The listing builds one solid part. Answer for the finished solid, in the listing's coordinates (mm). Round coordinates to 2 decimals unless told otherwise and drop trailing zeros. Write each loop counter-clockwise with the first axis right and the second up, starting at its lowest first coordinate (ties: lowest second). Pieces come first, ordered by that corner, then holes. Notation, with made-up numbers: M -34,13 L 2,13 A35 ccw 2,46 Z; hole C -23.75,53.25 d10. An arc over 180 degrees is marked long. One line per item, written item: value. Start each with the question number.
(1) Given P1, Ø1, axis at y = 2, z = -168, coming from the +X side; P2, Ø1.9, axis at x = 7.5, z = -222.3, coming from the +Y side; P3, Ø1.5, axis at x = 36, y = 2, coming from the +Z side, each flat-ended and moving along its own axis, determine where each tip first touches the part or whether it passes through.
(2) Consider probe 1 along Z at (x, y) = (145, 0.8); probe 2 along X at (y, z) = (2.15, -171.5); probe 3 along Z at (x, y) = (70, 2.45). Determine where each line is inside the solid, lowest interval first.
(3) For a pull along X with two mould halves and no side action, classify faces 1 (the cylindrical face through (3.01, 1.52, -2.85)), 2 (the cylindrical face through (167.15, 1.52, -3.01)), 3 (the flat face through (83, 3, -158)) as released by +X, released by -X, zero draft, split by the parting line, or undercut.
(4) Section C-C (y = 1.5) is taken. State how many separate pieces and enclosed holes the cut face has, plus the area to 3 significant figures.
(5) Section B-B (z = -149) is taken. Determine the outline of the cut face in (x, y).
(6) Section A-A (x = 179) is taken. Determine the outline of the cut face in (y, z).
```python
from build123d import *

# Parameters (mm, degrees)
BOSS_EXTRUDE1_DEPTH = 3
FILLET1_R           = 200
FILLET2_R           = 10
CUT_EXTRUDE2_DEPTH  = 429.345808882
SKETCH3_W           = 42
SKETCH3_H           = 23
SKETCH3_H_2         = 19
CUT_EXTRUDE3_DEPTH  = 429.345808882
SKETCH4_R           = 1.6
CUT_EXTRUDE5_DEPTH  = 429.345808882
SKETCH5_R           = 1.6
CUT_EXTRUDE6_DEPTH  = 429.345808882
SKETCH6_W           = 66
SKETCH6_H           = 15
SKETCH6_R           = 1.6
BOSS_EXTRUDE2_DEPTH = 3
FILLET3_R           = 5
SKETCH7_R           = 1.6
CUT_EXTRUDE7_DEPTH  = 435.224748243
SKETCH9_R           = 1.6
CUT_EXTRUDE8_DEPTH  = 435.224748243
SKETCH10_W          = 280
SKETCH10_H          = 108.680633212
CUT_EXTRUDE9_DEPTH  = 10


with BuildPart() as part:
    # Sketch1 → Boss-Extrude1 (new body)
    with BuildSketch(Plane(origin=(0, 0, 0), x_dir=(1, 0, 0), z_dir=(0, 1, 0))):
        Polygon((0, 0), (170, 0), (170, 300), (225, 300), (225, 367.51288694), (85, 330), (-55, 367.51288694), (-55, 300), (0, 300), align=None)
    extrude(amount=BOSS_EXTRUDE1_DEPTH)

    # Fillet1
    fillet1_edges = [part.edges().sort_by_distance(p)[0] for p in [
        (85, 1.5, -330),
    ]]
    fillet(fillet1_edges, radius=FILLET1_R)

    # Fillet2
    fillet2_edges = [part.edges().sort_by_distance(p)[0] for p in [
        (0, 1.5, -300),
        (-55, 1.5, -300),
        (-55, 1.5, -367.51288694),
        (225, 1.5, -367.51288694),
        (225, 1.5, -300),
        (170, 1.5, -300),
        (170, 1.5, 0),
        (0, 1.5, 0),
    ]]
    fillet(fillet2_edges, radius=FILLET2_R)

    # Sketch2 → Cut-Extrude2 (cut, through all)
    with BuildSketch(Plane(origin=(0, 3, 0), x_dir=(1, 0, 0), z_dir=(0, 1, 0))):
        with BuildLine():
            ThreePointArc((132.5, 80), (118.587572106, 113.587572106), (85, 127.5))
            Line((85, 127.5), (85, 32.5))
            ThreePointArc((85, 32.5), (118.587572106, 46.412427894), (132.5, 80))
        make_face()
        with BuildLine():
            Line((85, 32.5), (85, 127.5))
            ThreePointArc((85, 127.5), (37.5, 80), (85, 32.5))
        make_face()
    extrude(amount=-CUT_EXTRUDE2_DEPTH, mode=Mode.SUBTRACT)

    # Sketch3 → Cut-Extrude3 (cut, through all)
    with BuildSketch(Plane(origin=(0, 3, 0), x_dir=(1, 0, 0), z_dir=(0, 1, 0))):
        with Locations((40, 267.3)):
            Rectangle(SKETCH3_W, SKETCH3_H)
        with Locations((130, 267.3)):
            Rectangle(SKETCH3_W, SKETCH3_H)
        with Locations((40, 9.5)):
            Rectangle(SKETCH3_W, SKETCH3_H_2)
        with Locations((130, 9.5)):
            Rectangle(SKETCH3_W, SKETCH3_H_2)
    extrude(amount=-CUT_EXTRUDE3_DEPTH, mode=Mode.SUBTRACT)

    # Sketch4 → Cut-Extrude5 (cut, through all)
    with BuildSketch(Plane(origin=(0, 3, 0), x_dir=(1, 0, 0), z_dir=(0, 1, 0))):
        with Locations(Location((85, 133, 0), (0, 0, 270))):
            Circle(SKETCH4_R)
        with Locations(Location((122.476659403, 117.476659403, 0), (0, 0, 270))):
            Circle(SKETCH4_R)
        with Locations(Location((138, 80, 0), (0, 0, 270))):
            Circle(SKETCH4_R)
        with Locations(Location((122.476659403, 42.523340597, 0), (0, 0, 270))):
            Circle(SKETCH4_R)
        with Locations(Location((85, 27, 0), (0, 0, 270))):
            Circle(SKETCH4_R)
        with Locations(Location((47.523340597, 42.523340597, 0), (0, 0, 270))):
            Circle(SKETCH4_R)
        with Locations(Location((32, 80, 0), (0, 0, 270))):
            Circle(SKETCH4_R)
        with Locations(Location((47.523340597, 117.476659403, 0), (0, 0, 270))):
            Circle(SKETCH4_R)
    extrude(amount=-CUT_EXTRUDE5_DEPTH, mode=Mode.SUBTRACT)

    # Sketch5 → Cut-Extrude6 (cut, through all)
    with BuildSketch(Plane(origin=(0, 3, 0), x_dir=(1, 0, 0), z_dir=(0, 1, 0))):
        with Locations(Location((7.5, 312, 0), (0, 0, 270))):
            Circle(SKETCH5_R)
        with Locations(Location((7.5, 267.3, 0), (0, 0, 270))):
            Circle(SKETCH5_R)
        with Locations(Location((7.5, 222.3, 0), (0, 0, 270))):
            Circle(SKETCH5_R)
        with Locations(Location((7.5, 97.5, 0), (0, 0, 270))):
            Circle(SKETCH5_R)
        with Locations(Location((7.5, 7.5, 0), (0, 0, 270))):
            Circle(SKETCH5_R)
        with Locations(Location((7.5, 52.5, 0), (0, 0, 270))):
            Circle(SKETCH5_R)
        with Locations(Location((70, 7.5, 0), (0, 0, 270))):
            Circle(SKETCH5_R)
        with Locations(Location((100, 7.5, 0), (0, 0, 270))):
            Circle(SKETCH5_R)
        with Locations(Location((162.5, 7.5, 0), (0, 0, 270))):
            Circle(SKETCH5_R)
        with Locations(Location((162.5, 52.5, 0), (0, 0, 270))):
            Circle(SKETCH5_R)
        with Locations(Location((162.5, 97.5, 0), (0, 0, 270))):
            Circle(SKETCH5_R)
        with Locations(Location((162.5, 222.3, 0), (0, 0, 270))):
            Circle(SKETCH5_R)
        with Locations(Location((162.5, 267.3, 0), (0, 0, 270))):
            Circle(SKETCH5_R)
        with Locations(Location((162.5, 312, 0), (0, 0, 270))):
            Circle(SKETCH5_R)
        with Locations(Location((162.5, 342.75495241, 0), (0, 0, 270))):
            Circle(SKETCH5_R)
        with Locations(Location((109.337835254, 328.510193298, 0), (0, 0, 270))):
            Circle(SKETCH5_R)
        with Locations(Location((60.662164746, 328.510193298, 0), (0, 0, 270))):
            Circle(SKETCH5_R)
        with Locations(Location((7.5, 342.75495241, 0), (0, 0, 270))):
            Circle(SKETCH5_R)
        with Locations(Location((70, 267.5, 0), (0, 0, 270))):
            Circle(SKETCH5_R)
        with Locations(Location((100, 267.5, 0), (0, 0, 270))):
            Circle(SKETCH5_R)
    extrude(amount=-CUT_EXTRUDE6_DEPTH, mode=Mode.SUBTRACT)

    # Sketch6 → Boss-Extrude2 (add)
    # profile 1 of 2: a face of its own
    with BuildSketch(Plane.XZ):
        with Locations((-33, -52.5)):
            Rectangle(SKETCH6_W, SKETCH6_H)
        with Locations(Location((-45, -52.5, 0), (0, 0, 270))):
            Circle(SKETCH6_R, mode=Mode.SUBTRACT)
        with Locations(Location((-21, -52.5, 0), (0, 0, 270))):
            Circle(SKETCH6_R, mode=Mode.SUBTRACT)
    # profile 2 of 2: a face of its own
    with BuildSketch(Plane.XZ):
        with Locations((203, -52.5)):
            Rectangle(SKETCH6_W, SKETCH6_H)
        with Locations(Location((191, -52.5, 0), (0, 0, 270))):
            Circle(SKETCH6_R, mode=Mode.SUBTRACT)
        with Locations(Location((215, -52.5, 0), (0, 0, 270))):
            Circle(SKETCH6_R, mode=Mode.SUBTRACT)
    extrude(amount=-BOSS_EXTRUDE2_DEPTH)

    # Fillet3
    fillet3_edges = [part.edges().sort_by_distance(p)[0] for p in [
        (19, 1.5, 0),
        (61, 1.5, 0),
        (109, 1.5, 0),
        (109, 1.5, -19),
        (151, 1.5, -19),
        (151, 1.5, 0),
        (0, 1.5, -45),
        (0, 1.5, -60),
        (-66, 1.5, -60),
        (-66, 1.5, -45),
        (170, 1.5, -60),
        (170, 1.5, -45),
        (236, 1.5, -45),
        (236, 1.5, -60),
    ]]
    fillet(fillet3_edges, radius=FILLET3_R)

    # Sketch7 → Cut-Extrude7 (cut, through all)
    with BuildSketch(Plane(origin=(0, 3, 0), x_dir=(1, 0, 0), z_dir=(0, 1, 0))):
        with Locations(Location((130, 171.5, 0), (0, 0, 270))):
            Circle(SKETCH7_R)
        with Locations(Location((145, 171.5, 0), (0, 0, 270))):
            Circle(SKETCH7_R)
        with Locations(Location((145, 159.5, 0), (0, 0, 270))):
            Circle(SKETCH7_R)
        with Locations(Location((130, 159.5, 0), (0, 0, 270))):
            Circle(SKETCH7_R)
        with Locations(Location((25, 171.5, 0), (0, 0, 270))):
            Circle(SKETCH7_R)
        with Locations(Location((40, 171.5, 0), (0, 0, 270))):
            Circle(SKETCH7_R)
        with Locations(Location((40, 159.5, 0), (0, 0, 270))):
            Circle(SKETCH7_R)
        with Locations(Location((25, 159.5, 0), (0, 0, 270))):
            Circle(SKETCH7_R)
        with Locations(Location((70, 242, 0), (0, 0, 270))):
            Circle(SKETCH7_R)
        with Locations(Location((100, 242, 0), (0, 0, 270))):
            Circle(SKETCH7_R)
    extrude(amount=-CUT_EXTRUDE7_DEPTH, mode=Mode.SUBTRACT)

    # Sketch9 → Cut-Extrude8 (cut, through all)
    with BuildSketch(Plane(origin=(0, 3, 0), x_dir=(1, 0, 0), z_dir=(0, 1, 0))):
        with Locations(Location((-45, 307.5, 0), (0, 0, 270))):
            Circle(SKETCH9_R)
        with Locations(Location((-15, 307.5, 0), (0, 0, 270))):
            Circle(SKETCH9_R)
        with Locations(Location((-45, 327.5, 0), (0, 0, 270))):
            Circle(SKETCH9_R)
        with Locations(Location((-15, 327.5, 0), (0, 0, 270))):
            Circle(SKETCH9_R)
        with Locations(Location((185, 307.5, 0), (0, 0, 90))):
            Circle(SKETCH9_R)
        with Locations(Location((185, 327.5, 0), (0, 0, 90))):
            Circle(SKETCH9_R)
        with Locations(Location((215, 307.5, 0), (0, 0, 90))):
            Circle(SKETCH9_R)
        with Locations(Location((215, 327.5, 0), (0, 0, 90))):
            Circle(SKETCH9_R)
    extrude(amount=-CUT_EXTRUDE8_DEPTH, mode=Mode.SUBTRACT)

    # Sketch10 → Cut-Extrude9 (cut)
    with BuildSketch(Plane(origin=(0, 3, 0), x_dir=(1, 0, 0), z_dir=(0, 1, 0))):
        with Locations((85, 310.140316606)):
            Rectangle(SKETCH10_W, SKETCH10_H)
    extrude(amount=-CUT_EXTRUDE9_DEPTH, mode=Mode.SUBTRACT)


solid = part.part
```
Recorded:
1. P1: stops at x = 170
1. P2: passes through
1. P3: stops at z = -19
2. probe 1: z = -255.8 to -173.1, -169.9 to -161.1, -157.9 to -19
2. probe 2: x = 0 to 23.4, 26.6 to 38.4, 41.6 to 128.4, 131.6 to 143.4, 146.6 to 170
2. probe 3: z = -255.8 to -243.6, -240.4 to -125.07, -34.93 to -9.1, -5.9 to 0
3. face 1: released by -X
3. face 2: released by +X
3. face 3: zero draft
4. separate pieces: 1
4. enclosed holes: 33
4. area: 36,500 mm2
5. outline: M 0,0 L 170,0 L 170,3 L 0,3 Z
6. outline: M 0,-60 L 3,-60 L 3,-45 L 0,-45 Z
